Part model, mm, in its own coordinate system. A direction names the side the tool comes from. Coordinates: 2 decimals unless noted, no trailing zeros. Order: outer loops, then holes, each group sorted by start corner. A loop starts at its lowest first (then second) coordinate and runs counter-clockwise, first axis right, second up.
1) Tool access for faces 1 (the flat face through (0, 0, 18)), 2 (the flat face through (2.5, 0, 12)): list every direction of +Z, -Z, +X, -X, +Y, -Y with a clear straight run to the whole face (end or side of a thin tool).
2) Cut at A-A (z = 10.25). List the corners of the cut face in (x, y), and give its area (3 significant figures).
3) Pin check, flat tip, straight feed: pin 1 Ø1 at (y, z) = (0, 13.5) entering from +X. Stop position of the tip, or through.
4) Wall check: L1, parallel to Z at x = 2.75, y = -0.55; L2, parallel to Y at x = -0.5, z = 9.5; L3, parallel to X at y = -1.3, z = 10. Give the ranges that are in metal, low to high.
```python
from build123d import *

# Parameters (mm, degrees)
SKETCH1_R           = 3
BOSS_EXTRUDE1_DEPTH = 18
CUT_EXTRUDE1_START  = -12
CUT_EXTRUDE1_DEPTH  = 12
CHAMFER1_SIZE       = 0.5


with BuildPart() as part:
    # Sketch1 → Boss-Extrude1 (new body)
    with BuildSketch(Plane.XY):
        Circle(SKETCH1_R)
    extrude(amount=BOSS_EXTRUDE1_DEPTH)

    # Sketch2 → Cut-Extrude1 (cut)
    with BuildSketch(Plane.XY.offset(18).offset(CUT_EXTRUDE1_START)):
        with BuildLine():
            Line((2.5, 1.658312395), (2.5, -1.658312395))
            ThreePointArc((2.5, -1.658312395), (3, 0), (2.5, 1.658312395))
        make_face()
    extrude(amount=CUT_EXTRUDE1_DEPTH, mode=Mode.SUBTRACT)

    # Chamfer1
    chamfer1_edges = [part.edges().sort_by_distance(p)[0] for p in [
        (-3, 0, 18),
    ]]
    chamfer(chamfer1_edges, length=CHAMFER1_SIZE - 0.0001)  # a hair under: the kernel refuses the full size


solid = part.part
```
Geometry check:
1. face 1: +Z, +X, -X, +Y, -Y
1. face 2: +Z, +X, +Y, -Y
2. outline: (2.5, -1.66) - (2.5, 1.66) arc R3 ccw (long way) to start
2. area: 27.1 mm2
3. pin 1: stops at x = 2.5
4. L1: z = 0 to 6
4. L2: y = -2.96 to 2.96
4. L3: x = -2.7 to 2.5
